Autodesk Inventor part; units mm, degrees
ref_plane "YZ Plane" through (0, 0, 0) normal (1, 0, 0) x (0, 1, 0)
ref_plane "XZ Plane" through (0, 0, 0) normal (0, 1, 0) x (-1, 0, 0)
ref_plane "XY Plane" through (0, 0, 0) normal (0, 0, 1) x (1, 0, 0)
sketch "Szkic1" plane through (0, 0, 0) normal (0, 0, 1) x (1, 0, 0)
  line L0 (0, 0) -> (22, 0)
  line L1 (22, 0) -> (22, 13)
  line L2 (22, 13) -> (0, 13)
  line L3 (0, 13) -> (0, 0)
  dimension "d0" = 13
  dimension "d1" = 22
extrude "Wyciągnięcie proste1" add sketch "Szkic1" along normal blind 7
sketch "Szkic2" plane through (0, 0, 7) normal (0, 0, 1) x (1, 0, 0)
  line L0 (22, 0) -> (22, 13) construction
  line L1 (0, 13) -> (0, 0) construction
  line L2 (22, 0) -> (16.05, 0) construction
  line L3 (16.05, 0) -> (16.05, 13) construction
  line L4 (16.05, 13) -> (22, 13) construction
  line L5 (22, 13) -> (22, 0) construction
  line L6 (0, 0) -> (22, 0) construction
  line L7 (0, 0) -> (5.95, 0) construction
  line L8 (5.95, 0) -> (5.95, 13) construction
  line L9 (5.95, 13) -> (0, 13) construction
  line L10 (0, 13) -> (0, 0) construction
  line L11 (16.05, 0) -> (5.95, 0)
  line L12 (5.95, 0) -> (5.95, 13)
  line L13 (5.95, 13) -> (16.05, 13)
  line L14 (16.05, 13) -> (16.05, 0)
  dimension "d4" = 5.95
  dimension "d5" = 5.95
extrude "Wyciągnięcie proste2" cut sketch "Szkic2" against normal blind 4
fillet "Zaokrąglenie1" radius 3 2 edges at (16.05, 6.5, 3) (5.95, 6.5, 3)
sketch "Szkic3" plane through (0, 0, 7) normal (0, 0, 1) x (1, 0, 0)
  line L0 (0, 0) -> (22, 0) construction
  line L1 (0, 0) -> (0, 6.5) construction
  line L2 (0, 13) -> (0, 0) construction
  line L3 (0, 6.5) -> (22, 6.5) construction
  line L4 (22, 0) -> (22, 13) construction
  line L5 (0, 6.5) -> (2.975, 6.5) construction
  line L6 (22, 6.5) -> (19.025, 6.5) construction
  circle A0 centre (2.975, 6.5) radius 1.55
  circle A1 centre (19.025, 6.5) radius 1.55
  dimension "d9" = 2.975
  dimension "d10" = 2.975
  dimension "d11" = 3.1
  dimension "d12" = 3.1
extrude "Wyciągnięcie proste3" cut sketch "Szkic3" against normal blind 7
equation "\"d12\" = d11"
properties part number "Uchwyt_na_silnik"
The listing builds one solid part. Answer for the finished solid, in the listing's coordinates (mm). A direction names the side the tool comes from. Round coordinates to 2 decimals unless told otherwise and drop trailing zeros. Order: outer loops, then holes, each group sorted by start corner. A loop starts at its lowest first (then second) coordinate and runs counter-clockwise, first axis right, second up. Notation, with made-up numbers: (74, 33) -> (109, 33) arc R20 cw to (109, 59) -> close; hole circle Ø10 at (-29, 71.25). An arc over 180 degrees is marked (long way). Answer as CSV lines item,"result". Start each with the question number.
(1) Flat-ended cylindrical pins translate along their axes: pin 1 Ø1.2 at (x, y) = (11, 5.5) entering from +Z; pin 2 Ø1.5 at (y, z) = (5.5, 4.5) entering from -X. Find the tip coordinate at first contact, or state that the pin passes through.
(2) The part is cut by section B-B (y = 6.5). Determine the outline of the cut face in (x, z) (3 decimals), then the cut area to 3 significant figures.
(3) The part is cut by section D-D (y = 10.75). Determine the outline of the cut face in (x, z).
(4) Find the intervals of material crossed by probe 1 along X at (y, z) = (1.75, 6.5); probe 2 along Y at (x, z) = (2.75, 3); probe 3 along Y at (x, z) = (2.25, 6.25), in increasing order. Write a range as from..to.
(5) The part is cut by section C-C (z = 1.75). Determine the outline of the cut face in (x, y) (3 decimals).
(6) The part is cut by section A-A (z = 3.75). Determine the outline of the cut face in (x, y) (3 decimals), then the cut area to 3 significant figures.
(7) For a pull along X with two mould halves and no side action, classify faces 3 (the face through (11, 7, 3)), 4 (the face through (4.45, 6.97, 3.55)), 5 (the face through (2, 8, 7)), 6 (the face through (0, 7, 3)) as +X half, -X half, draft (parallel to the pull), parting line (faces both ways), or undercut.
(8) A tool of negligible diameter and unlimited length cuts with its end or side. For faces 1 (the face through (15.15, 6.41, 3.86)), 2 (the face through (18, 8, 7)), from which of +Z, -Z, +X, -X, +Y, -Y can it reach the whole face along a straight path? Write none if from no direction.
Evaluation:
1,pin 1,"z = 3"
1,pin 2,"x = 0"
2,outline,"(0, 0) -> (1.425, 0) -> (1.425, 7) -> (0, 7) -> close; (4.525, 0) -> (17.475, 0) -> (17.475, 7) -> (16.05, 7) -> (16.05, 6) arc R3 cw to (13.05, 3) -> (8.95, 3) arc R3 cw to (5.95, 6) -> (5.95, 7) -> (4.525, 7) -> close; (20.575, 0) -> (22, 0) -> (22, 7) -> (20.575, 7) -> close"
2,area,"74.1 mm²"
3,outline,"(0, 0) -> (22, 0) -> (22, 7) -> (16.05, 7) -> (16.05, 6) arc R3 cw to (13.05, 3) -> (8.95, 3) arc R3 cw to (5.95, 6) -> (5.95, 7) -> (0, 7) -> close"
4,probe 1,"0..5.95, 16.05..22"
4,probe 2,"0..4.97, 8.03..13"
4,probe 3,"0..5.13, 7.87..13"
5,outline,"(0, 0) -> (22, 0) -> (22, 13) -> (0, 13) -> close; hole circle Ø3.1 at (2.975, 6.5); hole circle Ø3.1 at (19.025, 6.5)"
6,outline,"(0, 0) -> (6.966, 0) -> (6.966, 13) -> (0, 13) -> close; (15.034, 0) -> (22, 0) -> (22, 13) -> (15.034, 13) -> close; hole circle Ø3.1 at (2.975, 6.5); hole circle Ø3.1 at (19.025, 6.5)"
6,area,"166 mm²"
7,face 3,"undercut"
7,face 4,"undercut"
7,face 5,"draft"
7,face 6,"-X half"
8,face 1,"+Z, +Y, -Y"
8,face 2,"+Z, +X, -X, +Y, -Y"
